from build123d import *

# Parameters (mm, degrees)
F1_DEPTH = 20
F2_R     = 5.25
F3_DEPTH = 6
F5_DEPTH = 7
F6_R     = 2.75
F7_DEPTH = 58.001


with BuildPart() as f1:
    # F0 (on Top) → F1 (new body)
    with BuildSketch(Plane.XY):
        with BuildLine():
            ThreePointArc((-5, 0), (-8.535534, 1.464466), (-10, 5))
            Line((-10, 5), (-10, 20))
            ThreePointArc((-10, 20), (-8.535534, 23.535534), (-5, 25))
            Line((-5, 25), (51, 25))
            ThreePointArc((51, 25), (54.535534, 23.535534), (56, 20))
            Line((56, 20), (56, 5))
            ThreePointArc((56, 5), (54.535534, 1.464466), (51, 0))
            Line((51, 0), (51, -3))
            ThreePointArc((51, -3), (56.656854, -0.656854), (59, 5))
            Line((59, 5), (59, 20))
            ThreePointArc((59, 20), (56.656854, 25.656854), (51, 28))
            Line((51, 28), (51, 40))
            ThreePointArc((51, 40), (56.656854, 42.343146), (59, 48))
            Line((59, 48), (59, 63))
            ThreePointArc((59, 63), (56.656854, 68.656854), (51, 71))
            Line((51, 71), (51, 68))
            ThreePointArc((51, 68), (54.535534, 66.535534), (56, 63))
            Line((56, 63), (56, 48))
            ThreePointArc((56, 48), (54.535534, 44.464466), (51, 43))
            Line((51, 43), (-5, 43))
            ThreePointArc((-5, 43), (-8.535534, 44.464466), (-10, 48))
            Line((-10, 48), (-10, 63))
            ThreePointArc((-10, 63), (-8.535534, 66.535534), (-5, 68))
            Line((-5, 68), (0, 68))
            Line((0, 68), (0, 71))
            Line((0, 71), (-5, 71))
            ThreePointArc((-5, 71), (-10.656854, 68.656854), (-13, 63))
            Line((-13, 63), (-13, 48))
            ThreePointArc((-13, 48), (-10.656854, 42.343146), (-5, 40))
            Line((-5, 40), (-5, 28))
            ThreePointArc((-5, 28), (-10.656854, 25.656854), (-13, 20))
            Line((-13, 20), (-13, 5))
            ThreePointArc((-13, 5), (-10.656854, -0.656854), (-5, -3))
            Line((-5, -3), (0, -3))
            Line((0, -3), (0, 0))
            Line((0, 0), (-5, 0))
        make_face()
    extrude(amount=F1_DEPTH)

    # F2 (on face) → F3 (cut)
    with BuildSketch(Plane(origin=(-5, 0, 0), x_dir=(0, -1, 0), z_dir=(-1, 0, 0))):
        with Locations((-34, 10)):
            Circle(F2_R)
    extrude(amount=-F3_DEPTH, mode=Mode.SUBTRACT)

    # F4 (on face) → F5 (cut)
    with BuildSketch(Plane.YZ.offset(51)):
        Polygon((38, 7.690599), (38, 12.309401), (34, 14.618802), (30, 12.309401), (30, 7.690599), (34, 5.381198), align=None)
    extrude(amount=-F5_DEPTH, mode=Mode.SUBTRACT)

    # F6 (on face) → F7 (cut, through all)
    with BuildSketch(Plane(origin=(1, 0, 0), x_dir=(0, -1, 0), z_dir=(-1, 0, 0))):
        with Locations((-34, 10)):
            Circle(F6_R)
    extrude(amount=-F7_DEPTH, mode=Mode.SUBTRACT)


solid = f1.part
Geometry check sheet. Reference: the model listing, model coordinates, mm. A direction names the side the tool comes from. Round coordinates to 2 decimals unless told otherwise and drop trailing zeros. Order: outer loops, then holes, each group sorted by start corner. A loop starts at its lowest first (then second) coordinate and runs counter-clockwise, first axis right, second up. Notation, with made-up numbers: M -28.5,-25.75 L 25.5,-25.75 A9 cw 25.5,-15.75 Z; hole C 56,39.5 d1. An arc over 180 degrees is marked long. Write each question's results on one line, items separated by ' | '. Start each with the question number.
1. Cross-section at C-C on x = 53.5. Record the boundary of the cut face in (y, z).
2. Go/stop test with flat-tipped pins: P1, Ø2.5, axis at x = 46, z = 9, coming from the +Y side; P2, Ø3.5, axis at y = 69.5, z = 12, coming from the +X side; P3, Ø0.9, axis at y = -1, z = 6.5, coming from the +X side; P4, Ø3.5, axis at y = 34, z = 10, coming from the -X side. Record where each tip stops, or that it passes through.
3. Cross-section at D-D on y = 46. Record the boundary of the cut face in (x, z), plus the area to 3 significant figures.
4. Draft check along X on faces 4 (the face through (-10.594, 25.719, 9.86)), 5 (the face through (-3, -3, 10)), 6 (the face through (-3, 68, 10)), 7 (the face through (-10, 55, 10)). Enter one of: pulls with the +X half, pulls with the -X half, needs draft (parallel to the pull), parting line crosses it, or undercut.
5. Set-up check for faces 1 (the face through (-2.04, 37.87, 13.55)), 2 (the face through (48, 38, 10)), 3 (the face through (-2, 0, 10)): record each of +Z, -Z, +X, -X, +Y, -Y from which the full face is reachable in a straight line by a thin tool's end or side.
6. Cross-section at A-A on x = 8. Record the boundary of the cut face in (y, z), plus the area to 3 significant figures.
7. Material ranges on L1, parallel to Z at x = -1, y = 34; L2, parallel to X at y = 60, z = 11.75; L3, parallel to Z at x = 13, y = 34, recorded low to high. Write a range as from..to.
8. Cross-section at B-B on y = 14. Record the boundary of the cut face in (x, z), plus the area to 3 significant figures.
Resolved:
1) outline: M -2.6,0 L 0.67,0 L 0.67,20 L -2.6,20 Z; M 24.33,0 L 27.6,0 L 27.6,20 L 24.33,20 Z; M 40.4,0 L 43.67,0 L 43.67,20 L 40.4,20 Z; M 67.33,0 L 70.6,0 L 70.6,20 L 67.33,20 Z
2) P1: y = 43 | P2: x = 57.44 | P3: x = 56.76 | P4: through
3) outline: M -12.75,0 L -9.58,0 L -9.58,20 L -12.75,20 Z; M 55.58,0 L 58.75,0 L 58.75,20 L 55.58,20 Z | area: 127 mm2
4) face 4: pulls with the -X half | face 5: needs draft | face 6: undercut | face 7: undercut
5) face 1: -X | face 2: +X | face 3: +Z, -Z
6) outline: M 25,0 L 43,0 L 43,20 L 25,20 Z; hole C 34,10 d5.5 | area: 336 mm2
7) L1: 0..4.75, 15.25..20 | L2: -13..-10, 56..59 | L3: 0..7.25, 12.75..20
8) outline: M -13,0 L -10,0 L -10,20 L -13,20 Z; M 56,0 L 59,0 L 59,20 L 56,20 Z | area: 120 mm2
